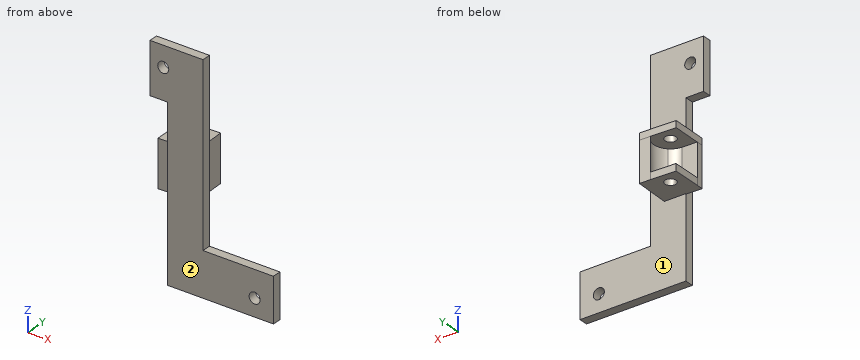
from build123d import *

# Parameters (mm, degrees)
BOSS_EXTRUDE2_DEPTH = 23.061761584
BOSS_EXTRUDE3_START = -4.011761584
SKETCH5_R           = 3.175
BOSS_EXTRUDE3_DEPTH = 4.011761584
BOSS_EXTRUDE5_START = 3.81
SKETCH6_R           = 3.175
BOSS_EXTRUDE5_DEPTH = 3.81
SKETCH7_R           = 3.175
BOSS_EXTRUDE6_DEPTH = 5.08


with BuildPart() as part:
    # Sketch1 → Boss-Extrude2 (new body)
    with BuildSketch(Plane.XY):
        with BuildLine():
            Line((346.486451601, 100.481133449), (337.915550261, 100.173402481))
            Line((337.915550261, 100.173402481), (338.052257003, 96.365855861))
            Line((338.052257003, 96.365855861), (359.243555017, 97.126711503))
            Line((359.243555017, 97.126711503), (358.508072741, 117.611312321))
            Line((358.508072741, 117.611312321), (352.162161707, 117.383467749))
            ThreePointArc((352.162161707, 117.383467749), (355.663551295, 110.341766857), (352.67617906, 103.067092457))
            ThreePointArc((352.67617906, 103.067092457), (349.816499797, 101.211177598), (346.486451601, 100.481133449))
        make_face()
    extrude(amount=-BOSS_EXTRUDE2_DEPTH)

    # Sketch5 → Boss-Extrude3 (add)
    with BuildSketch(Plane(origin=(0, 0, -23.061761584), x_dir=(-1, 0, 0), z_dir=(0, 0, -1)).offset(BOSS_EXTRUDE3_START)):
        with BuildLine():
            Line((-337.915550261, 116.871955208), (-337.915550261, 100.173402481))
            Line((-337.915550261, 100.173402481), (-346.486451601, 100.481133449))
            ThreePointArc((-346.486451601, 100.481133449), (-355.174204205, 106.967937449), (-352.162161707, 117.383467749))
            Line((-352.162161707, 117.383467749), (-337.915550261, 116.871955208))
        make_face()
        with Locations((-346.144684744, 110)):
            Circle(SKETCH5_R, mode=Mode.SUBTRACT)
    extrude(amount=BOSS_EXTRUDE3_DEPTH)

    # Sketch6 → Boss-Extrude5 (add)
    with BuildSketch(Plane.XY.offset(BOSS_EXTRUDE5_START)):
        Polygon((337.780813741, 116.867117607), (338.052257003, 96.365855861), (359.243555017, 97.126711503), (358.508072741, 117.611312321), align=None)
        with Locations(Location((346.144684744, 110, 0), (0, 0, 180))):
            Circle(SKETCH6_R, mode=Mode.SUBTRACT)
    extrude(amount=-BOSS_EXTRUDE5_DEPTH)

    # Sketch7 → Boss-Extrude6 (add)
    with BuildSketch(Plane(origin=(0, 97.126711503, 0), x_dir=(1, 0, 0), z_dir=(0, 1, 0))):
        Polygon((367.184506183, -32.004), (367.184506183, -57.404), (336.704506183, -57.404), (336.704506183, -27.94), (346.864506183, -27.94), (346.864506183, 44.958), (346.864506183, 69.596), (407.824506183, 69.596), (407.824506183, 44.196), (367.184506183, 44.196), align=None)
        with Locations(Location((396.977487406, 59.456782771, 0), (0, 0, 270))):
            Circle(SKETCH7_R, mode=Mode.SUBTRACT)
        with Locations(Location((344.324506183, -45.552790878, 0), (0, 0, 270))):
            Circle(SKETCH7_R, mode=Mode.SUBTRACT)
    extrude(amount=-BOSS_EXTRUDE6_DEPTH)


solid = part.part
Design review of the part built by this model. Coordinates are the model's own, in mm. Face numbers are marked on the shaded views. Give positions to 0.01 mm unless a question says otherwise; leave off trailing zeros. Order: outer loops, then holes, each group sorted by start corner. A loop starts at its lowest first (then second) coordinate and runs counter-clockwise, first axis right, second up. Notation, with made-up numbers: (51.5, 87.5) - (87.5, 87.5) arc R27 cw to (87.5, 117.5) - close; hole circle Ø4 at (51.25, 28.5). An arc over 180 degrees is marked (long way). Write item = value, one per line. Start each with the question number.
Q1. We need section A-A on y = 110. State the section outline as (x, z) points.
Q2. Mouldability with a two-part tool opening along Y and no side actions: class the marked faces 1 and 2 as released by +Y, released by -Y, zero draft, split by the parting line, or undercut.
Q3. Clearance check with flat-ended pins moving along their axes: pin 1 Ø5.5 at (x, y) = (341.5, 95.5) entering from -Z; pin 2 Ø4.5 at (y, z) = (109.5, -20.5) entering from -X; pin 3 Ø1.5 at (x, y) = (389.5, 93.5) entering from +Z. State where each tip first meets the part, or that it passes through.
Q4. To check wall thickness, follow L1, parallel to Z at x = 349.5, y = 115.5; L2, parallel to Z at x = 358.5, y = 102.5; L3, parallel to Y at x = 357.5, z = 35.5. State the ranges of each line that lie inside material, in increasing order. Write a range as from..to.
Q5. We need section C-C on y = 95. State how many separate pieces and enclosed holes the cut face has, plus the area to 3 significant figures.
Q6. We need section B-B on z = -58. State the section outline as (x, y) points, plus the area to 3 significant figures.
Q7. We need section D-D on x = 386. State the section outline as (y, z) points, plus the area to 3 significant figures.
Working result:
q1.outline = (337.87, 0) - (342.97, 0) - (342.97, 3.81) - (337.87, 3.81) - close; (337.92, -23.06) - (342.97, -23.06) - (342.97, -19.05) - (337.92, -19.05) - close; (349.32, -23.06) - (358.78, -23.06) - (358.78, 3.81) - (349.32, 3.81) - (349.32, 0) - (355.67, 0) - (355.67, -19.05) - (349.32, -19.05) - close
q2.face_1 = released by +Y
q2.face_2 = released by -Y
q3.pin_1 = -23.06
q3.pin_2 = 337.92
q3.pin_3 = -44.2
q4.L1 = -23.06..-19.05, 0..3.81
q4.L2 = -23.06..3.81
q4.L3 = 92.05..97.13
q5.separate_pieces = 1
q5.enclosed_holes = 2
q5.area = 3,850 mm²
q6.outline = (346.86, 92.05) - (394.16, 92.05) - (394.16, 97.13) - (346.86, 97.13) - close; (399.8, 92.05) - (407.82, 92.05) - (407.82, 97.13) - (399.8, 97.13) - close
q6.area = 281 mm²
q7.outline = (92.05, -69.6) - (97.13, -69.6) - (97.13, -44.2) - (92.05, -44.2) - close
q7.area = 129 mm²
